from build123d import *

# Parameters (mm, degrees)
SKETCH_R     = 6
PAD_DEPTH    = 5.8
SKETCH001_R  = 4.5
PAD001_DEPTH = 7
SKETCH002_W  = 0.6
SKETCH002_H  = 12
POCKET_DEPTH = 6
SKETCH003_R  = 0.4
PAD002_DEPTH = 5
SKETCH004_W  = 3.6
SKETCH004_H  = 11.44727
PAD003_DEPTH = 1.5


with BuildPart() as part:
    # Sketch → Pad (new body)
    with BuildSketch(Plane.XY):
        Circle(SKETCH_R)
    extrude(amount=PAD_DEPTH)

    # Sketch001 → Pad001 (new body)
    with BuildSketch(Plane.XY.offset(5.8)):
        Circle(SKETCH001_R)
    extrude(amount=PAD001_DEPTH)

    # Sketch002 → Pocket (cut)
    with BuildSketch(Plane.XY.offset(5.8)):
        with Locations((-5.7, 0)):
            Rectangle(SKETCH002_W, SKETCH002_H)
    extrude(amount=-POCKET_DEPTH, mode=Mode.SUBTRACT)

    # Sketch003 → Pad002 (new body)
    with BuildSketch(Plane(origin=(0, 0, 0), x_dir=(1, 0, 0), z_dir=(0, 0, -1))):
        with Locations((-2.5, 2.5)):
            Circle(SKETCH003_R)
        with Locations((2.5, 2.5)):
            Circle(SKETCH003_R)
        with Locations((-2.5, -2.5)):
            Circle(SKETCH003_R)
        with Locations((2.5, -2.5)):
            Circle(SKETCH003_R)
    extrude(amount=PAD002_DEPTH)

    # Sketch004 → Pad003 (new body)
    with BuildSketch(Plane(origin=(0, 0, 0), x_dir=(1, 0, 0), z_dir=(0, 0, -1))):
        Rectangle(SKETCH004_W, SKETCH004_H)
    extrude(amount=PAD003_DEPTH)


solid = part.part
Check sheet for the modelled part. Datum: model origin and axes. Units: mm. A direction names the side the tool comes from. Round coordinates to 2 decimals unless told otherwise and drop trailing zeros. Loops run counter-clockwise (first coordinate to the right, second up) from the corner with the lowest first, then second, coordinate; pieces in that order, holes last. Notation, with made-up numbers: (-20, 26) -> (8, 26) arc R20 ccw to (8, 39) -> close; hole circle Ø2 at (-33.5, 47). An arc over 180 degrees is marked (long way). Put each result on its own line as item: value. Start each with the question number.
1. Scan lines: probe 1 along Z at (x, y) = (-2, 0.25); probe 2 along Y at (x, z) = (2.5, -1.25); probe 3 along X at (y, z) = (1, -0.25). Record each from-to range of solid material in increasing order.
2. Draft check along X on faces 1 (the face through (0, 0, 12.8)), 2 (the face through (-5.4, 0, 3)), 3 (the face through (1.8, 0, -1)). Enter one of: +X half, -X half, draft (parallel to the pull), parting line (faces both ways), or undercut.
3. Section check A-A (z = -0.5). Enter the section's corners in (x, y), plus the area to 3 significant figures.
4. Section check C-C (y = 0.5). Enter the section's corners in (x, z), plus the area to 3 significant figures.
5. Gauge pin test, flat ends, axial feed: pin 1 (3 mm diameter, centred on x = -0.5, z = 8.5, fed in from -Y); pin 2 (5 mm diameter, centred on y = -1, z = 4.5, fed in from +X); pin 3 (1.1 mm diameter, centred on x = -3.5, y = 2, fed in from -Z); pin 4 (1.8 mm diameter, centred on x = 1, y = 1.5, fed in from -Z). Record the tip position at first contact, or that the pin passes through.
6. Section check B-B (x = 0). Enter the section's corners in (y, z), plus the area to 3 significant figures.
7. Access from +Z, -Z, +X, -X, +Y, -Y to the whole of each face (thin tool, end or side, straight path). Record for faces 4 (the face through (-0.59, 4.46, 9.25)), 5 (the face through (0, 5.724, -1)), 6 (the face through (-1.8, 0, -1)).
8. Section check D-D (z = -3.5). Enter the section's corners in (x, y).
Findings:
1. probe 1: z = 0 to 12.8
1. probe 2: y = -2.9 to -2.1, 2.1 to 2.9
1. probe 3: x = -1.8 to 1.8
2. face 1: draft
2. face 2: -X half
2. face 3: undercut
3. outline: circle Ø0.8 at (-2.5, -2.5); circle Ø0.8 at (-2.5, 2.5); (-1.8, -5.72) -> (1.8, -5.72) -> (1.8, 5.72) -> (-1.8, 5.72) -> close; circle Ø0.8 at (2.5, -2.5); circle Ø0.8 at (2.5, 2.5)
3. area: 43.2 mm^2
4. outline: (-5.4, 0) -> (-1.8, 0) -> (-1.8, -1.5) -> (1.8, -1.5) -> (1.8, 0) -> (5.98, 0) -> (5.98, 5.8) -> (4.47, 5.8) -> (4.47, 12.8) -> (-4.47, 12.8) -> (-4.47, 5.8) -> (-5.4, 5.8) -> close
4. area: 134 mm^2
5. pin 1: stops at y = -4.5
5. pin 2: stops at x = 6
5. pin 3: stops at z = 0
5. pin 4: stops at z = -1.5
6. outline: (-6, 0) -> (-5.72, 0) -> (-5.72, -1.5) -> (5.72, -1.5) -> (5.72, 0) -> (6, 0) -> (6, 5.8) -> (4.5, 5.8) -> (4.5, 12.8) -> (-4.5, 12.8) -> (-4.5, 5.8) -> (-6, 5.8) -> close
6. area: 150 mm^2
7. face 4: +Z
7. face 5: -Z, +X, -X, +Y
7. face 6: -Z, +Y, -Y
8. outline: circle Ø0.8 at (-2.5, -2.5); circle Ø0.8 at (-2.5, 2.5); circle Ø0.8 at (2.5, -2.5); circle Ø0.8 at (2.5, 2.5)
